Source: CAD feature listing. Evaluate the final solid. Frame: model axes, mm. A direction names the side the tool comes from. Round coordinates to 2 decimals unless told otherwise and drop trailing zeros. Write each loop counter-clockwise with the first axis right and the second up, starting at its lowest first coordinate (ties: lowest second). Pieces come first, ordered by that corner, then holes. Notation, with made-up numbers: M 14.5,-21 L 23.5,-21 A12 cw 23.5,-14 Z; hole C 42.5,-5.5 d3. An arc over 180 degrees is marked long. Use a Markdown table: item, result.
```python
from build123d import *

# Parameters (mm, degrees)
F1_DEPTH = 63.5
F0_W     = 25.4
F0_H     = 19.05
F2_DEPTH = 25.4
F3_DEPTH = 7.9375


with BuildPart() as f1:
    # F0 (on Front) → F1 (new body, symmetric)
    with BuildSketch(Plane.XZ):
        Polygon((-41.275, -9.525), (41.275, -9.525), (41.275, 9.525), (22.225, 9.525), (-41.275, 9.525), align=None)
    extrude(amount=F1_DEPTH, both=True)

    # F0 (on Front) → F2 (join, symmetric)
    with BuildSketch(Plane.XZ):
        with BuildLine():
            Line((22.225, 9.525), (41.275, 9.525))
            Line((41.275, 9.525), (41.275, 31.427365057))
            ThreePointArc((41.275, 31.427365057), (44.6279932249, 39.5222067751), (52.722834943, 42.8752))
            Line((52.722834943, 42.8752), (57.6861744831, 42.8752))
            Line((57.6861744831, 42.8752), (57.6861744831, 61.9252))
            Line((57.6861744831, 61.9252), (52.722834943, 61.9252))
            ThreePointArc((52.722834943, 61.9252), (31.1576090433, 52.9925909567), (22.225, 31.427365057))
            Line((22.225, 31.427365057), (22.225, 9.525))
        make_face()
        with Locations((70.3861744831, 52.4002)):
            Rectangle(F0_W, F0_H)
    extrude(amount=F2_DEPTH, both=True)

    # F0 (on Front) → F3 (join, symmetric)
    with BuildSketch(Plane.XZ):
        with BuildLine():
            add(Edge.make_bspline(
                [(-41.275, 9.525), (-41.7181551456, 48.1705069542), (17.0384701341, 67.8877606988), (52.722834943, 61.9252)],
                knots=[0, 0, 0, 0, 107.6167920634, 107.6167920634, 107.6167920634, 107.6167920634], degree=3))
            Line((-41.275, 9.525), (22.225, 9.525))
            Line((22.225, 9.525), (22.225, 31.427365057))
            ThreePointArc((22.225, 31.427365057), (31.1576090433, 52.9925909567), (52.722834943, 61.9252))
        make_face()
    extrude(amount=F3_DEPTH, both=True)

    # F0 (on Front) → F4 (revolve)
    with BuildSketch(Plane.XZ):
        Polygon((83.0861744831, 66.675), (83.0861744831, 61.9252), (83.0861744831, 42.8752), (83.0861744831, 38.1), (108.4861744831, 38.1), (108.4861744831, 66.675), align=None)
    revolve(axis=Axis((83.0861744831, 0, 50.0126), (0, 0, 1)))


solid = f1.part
```
Q1. Section A-A on y = 11. Return loops of the section in (x, z) (3 decimals).
Results are:
| item | result |
|---|---|
| outline | M -41.275,-9.525 L 41.275,-9.525 L 41.275,31.427 A11.448 cw 52.723,42.875 L 60.192,42.875 L 60.192,38.1 L 105.981,38.1 L 105.981,66.675 L 60.192,66.675 L 60.192,61.925 L 52.723,61.925 A30.498 ccw 22.225,31.427 L 22.225,9.525 L -41.275,9.525 Z |
Q2. Section B-B on x = 63.5. Return loops of the section in (y, z) (3 decimals).
Results are:
| item | result |
|---|---|
| outline | M -25.4,42.875 L -16.172,42.875 L -16.172,38.1 L 16.172,38.1 L 16.172,42.875 L 25.4,42.875 L 25.4,61.925 L 16.172,61.925 L 16.172,66.675 L -16.172,66.675 L -16.172,61.925 L -25.4,61.925 Z |
Q3. Section C-C on z = 4. Return loops of the section in (x, y) (3 decimals), plus the area to 3 significant figures.
Results are:
| item | result |
|---|---|
| outline | M -41.275,-63.5 L 41.275,-63.5 L 41.275,63.5 L -41.275,63.5 Z |
| area | 10,500 mm^2 |
Q4. Reachability of faces 4 (the cylindrical face through (44.539, -0.356, 39.433)), 5 (the cylindrical face through (31.4, -16.79, 53.23)), 6 (the cylindrical face through (31.4, 16.55, 53.23)) from +Z, -Z, +X, -X, +Y, -Y: full face, straight path, thin tool, end or side. Return the list, or none.
Results are:
| item | result |
|---|---|
| face 4 | -Z, +Y, -Y |
| face 5 | +Z, -X, -Y |
| face 6 | +Z, -X, +Y |
Q5. Section D-D on y = -39. Return loops of the section in (x, z) (3 decimals), plus the area to 3 significant figures.
Results are:
| item | result |
|---|---|
| outline | M -41.275,-9.525 L 41.275,-9.525 L 41.275,9.525 L -41.275,9.525 Z |
| area | 1,570 mm^2 |
Q6. Mould query, pull axis X, two halves, no side actions, for faces 1 (the flat face through (57, 2, 61.925)), 2 (the flat face through (22.225, 17, 21)), 3 (the flat face through (83, 0, 38.1)). Classes: +X half, -X half, draft (parallel to the pull), parting line (faces both ways), or undercut.
Results are:
| item | result |
|---|---|
| face 1 | undercut |
| face 2 | -X half |
| face 3 | draft |
Q7. Line query: L1, parallel to Y at x = 13.5, z = 52.5; L2, parallel to Z at x = -1.5, y = -8 (3 decimals); L3, parallel to Y at x = 46.5, z = 42. Output: solid intervals per line, ascending.
Results are:
| item | result |
|---|---|
| L1 | -7.94 to 7.94 |
| L2 | -9.525 to 9.525 |
| L3 | -25.4 to 25.4 |
Q8. First-contact query: pin 1 Ø5 at (y, z) = (27.5, 1) entering from +X (3 decimals); pin 2 Ø8.5 at (y, z) = (-15.5, 25) entering from -X (3 decimals); pin 3 Ø15.5 at (x, z) = (53, 41) entering from +Y. Flat tips, straight axial feed; report the tip coordinate or a pass-through.
Results are:
| item | result |
|---|---|
| pin 1 | x = 41.275 |
| pin 2 | x = 22.225 |
| pin 3 | y = 25.4 |
